Geometry check sheet. Reference: the model listing, model coordinates, mm. A direction names the side the tool comes from. Give positions to 0.01 mm unless a question says otherwise; leave off trailing zeros. Loops run counter-clockwise (first coordinate to the right, second up) from the corner with the lowest first, then second, coordinate; pieces in that order, holes last. Notation, with made-up numbers: (23.25, -35) - (78.25, -35) arc R32 cw to (78.25, -5) - close; hole circle Ø1 at (-28, -28.5). An arc over 180 degrees is marked (long way). Use a Markdown table: item, result. Add a question column.
1. Draft check along X on faces 5 (the flat face through (100, 48, 26)), 6 (the flat face through (-10, 65, 147)), 7 (the flat face through (-1, 78, 200)). Enter one of: pulls with the +X half, pulls with the -X half, needs draft (parallel to the pull), parting line crosses it, or undercut.
2. Cross-section at A-A on y = -42.5. Enter the section's corners in (x, z), and give its area (3 significant figures).
3. Set-up check for faces 1 (the cylindrical face through (-2.17, 22.74, 7.54)), 2 (the flat face through (-95, 60, 28)), 3 (the cylindrical face through (-97.54, 53.61, 32.55)), 4 (the flat face through (13, 65, 143)): record each of +Z, -Z, +X, -X, +Y, -Y from which the full face is reachable in a straight line by a thin tool's end or side.
4. Cross-section at D-D on y = 32.5. Enter the section's corners in (x, z), and give its area (3 significant figures).
5. Depth check by flat-ended pin: P1, Ø10, axis at x = 59, y = 27.5, coming from the +Z side; P2, Ø4, axis at x = 41, y = -60, coming from the +Z side; P3, Ø10, axis at y = 60.5, z = 149, coming from the +X side. Enter the tip coordinate at first touch or a pass-through.
6. Cross-section at B-B on z = 176. Enter the section's corners in (x, y).
7. Cross-section at C-C on y = 5. Enter the section's corners in (x, z).
8. Material ranges on L1, parallel to Y at x = 0, z = 7; L2, parallel to X at y = 32, z = 6; L3, parallel to Z at x = 18, y = -58, recorded low to high.
from build123d import *

# Parameters (mm, degrees)
SKETCH_W      = 200
SKETCH_H      = 160
PAD_DEPTH     = 10
SKETCH001_R   = 7.5
SKETCH001_R_2 = 10
POCKET_DEPTH  = 5
SKETCH002_W   = 200
SKETCH002_H   = 5
PAD001_DEPTH  = 190
PAD002_DEPTH  = 5
PAD003_DEPTH  = 5
SKETCH005_W   = 3
SKETCH005_H   = 30
PAD004_DEPTH  = 20
PAD005_DEPTH  = 3


with BuildPart() as part:
    # Sketch → Pad (new body)
    with BuildSketch(Plane.XY):
        Rectangle(SKETCH_W, SKETCH_H)
    extrude(amount=PAD_DEPTH)

    # Sketch001 → Pocket (cut)
    with BuildSketch(Plane.XY.offset(10)):
        with Locations((57.5, 5)):
            Circle(SKETCH001_R)
        with Locations((0, 5)):
            Circle(SKETCH001_R)
        with Locations((-57.5, 5)):
            Circle(SKETCH001_R)
        with Locations((-57.5, 32.5)):
            Circle(SKETCH001_R_2)
        with Locations((0, 32.5)):
            Circle(SKETCH001_R_2)
        with Locations((57.5, 32.5)):
            Circle(SKETCH001_R_2)
        with BuildLine():
            ThreePointArc((-57.5, -15), (-85, -42.5), (-57.5, -70))
            Line((-57.5, -70), (57.5, -70))
            ThreePointArc((57.5, -70), (85, -42.5), (57.5, -15))
            Line((-57.5, -15), (57.5, -15))
        make_face()
    extrude(amount=-POCKET_DEPTH, mode=Mode.SUBTRACT)

    # Sketch002 → Pad001 (new body)
    with BuildSketch(Plane.XY.offset(10)):
        with Locations((0, 77.5)):
            Rectangle(SKETCH002_W, SKETCH002_H)
    extrude(amount=PAD001_DEPTH)

    # Sketch003 → Pad002 (new body)
    with BuildSketch(Plane.YZ.offset(100)):
        with BuildLine():
            Line((75, 10), (0, 10))
            ThreePointArc((0, 10), (53.033009, 31.966991), (75, 85))
            Line((75, 10), (75, 85))
        make_face()
    extrude(amount=-PAD002_DEPTH)

    # Sketch004 → Pad003 (new body)
    with BuildSketch(Plane(origin=(-100, 0, 0), x_dir=(0, -1, 0), z_dir=(-1, 0, 0))):
        with BuildLine():
            Line((-75, 10), (0, 10))
            ThreePointArc((-75, 85), (-53.033009, 31.966991), (0, 10))
            Line((-75, 10), (-75, 85))
        make_face()
    extrude(amount=-PAD003_DEPTH)

    # Sketch005 → Pad004 (new body)
    with BuildSketch(Plane.XZ.offset(-75)):
        with Locations((-11.5, 147)):
            Rectangle(SKETCH005_W, SKETCH005_H)
        with Locations((11.5, 147)):
            Rectangle(SKETCH005_W, SKETCH005_H)
    extrude(amount=PAD004_DEPTH)

    # Sketch006 → Pad005 (new body)
    with BuildSketch(Plane.YZ.offset(13)):
        with BuildLine():
            ThreePointArc((55, 132), (57.928932, 124.928932), (65, 122))
            ThreePointArc((74.999966, 111.999966), (72.071058, 119.071044), (65, 122))
            Line((75, 132), (74.999966, 111.999966))
            Line((55, 132), (75, 132))
        make_face()
    extrude(amount=-PAD005_DEPTH)


solid = part.part
Values found:
| question | item | result |
|---|---|---|
| 1 | face 5 | pulls with the +X half |
| 1 | face 6 | undercut |
| 1 | face 7 | needs draft |
| 2 | outline | (-100, 0) - (100, 0) - (100, 10) - (85, 10) - (85, 5) - (-85, 5) - (-85, 10) - (-100, 10) - close |
| 2 | area | 1,150 mm2 |
| 3 | face 1 | +Z |
| 3 | face 2 | +Z, -Y |
| 3 | face 3 | +Z, +X, -X, -Y |
| 3 | face 4 | +Z, +X, -Y |
| 4 | outline | (-100, 0) - (100, 0) - (100, 17.41) - (95, 17.41) - (95, 10) - (67.5, 10) - (67.5, 5) - (47.5, 5) - (47.5, 10) - (10, 10) - (10, 5) - (-10, 5) - (-10, 10) - (-47.5, 10) - (-47.5, 5) - (-67.5, 5) - (-67.5, 10) - (-95, 10) - (-95, 17.41) - (-100, 17.41) - close |
| 4 | area | 1,770 mm2 |
| 5 | P1 | stops at z = 10 |
| 5 | P2 | stops at z = 5 |
| 5 | P3 | stops at x = 13 |
| 6 | outline | (-100, 75) - (100, 75) - (100, 80) - (-100, 80) - close |
| 7 | outline | (-100, 0) - (100, 0) - (100, 10.17) - (95, 10.17) - (95, 10) - (65, 10) - (65, 5) - (50, 5) - (50, 10) - (7.5, 10) - (7.5, 5) - (-7.5, 5) - (-7.5, 10) - (-50, 10) - (-50, 5) - (-65, 5) - (-65, 10) - (-95, 10) - (-95, 10.17) - (-100, 10.17) - close |
| 8 | L1 | y = -80 to -70, -15 to -2.5, 12.5 to 22.5, 42.5 to 80 |
| 8 | L2 | x = -100 to -67.49, -47.51 to -9.99, 9.99 to 47.51, 67.49 to 100 |
| 8 | L3 | z = 0 to 5 |
